Build history of the part. All positions in model axes, mm. A direction names the side the tool comes from. Round coordinates to 2 decimals unless told otherwise and drop trailing zeros. Order: outer loops, then holes, each group sorted by start corner. A loop starts at its lowest first (then second) coordinate and runs counter-clockwise, first axis right, second up. Notation, with made-up numbers: M -25,16.25 L -7,16.25 A22 cw -7,24.25 Z; hole C 7,62 d5. An arc over 180 degrees is marked long. Use CSV: the item, a comma, the result in double quotes.
Autodesk Inventor part; units mm, degrees
ref_plane "YZ Plane" through (0, 0, 0) normal (1, 0, 0) x (0, 1, 0)
ref_plane "XZ Plane" through (0, 0, 0) normal (0, 1, 0) x (-1, 0, 0)
ref_plane "XY Plane" through (0, 0, 0) normal (0, 0, 1) x (1, 0, 0)
sketch "Skizze1" plane through (0, 0, 0) normal (0, 0, 1) x (1, 0, 0)
  line L0 (0, 9.6853) -> (0, -8.6142)
  line L1 (-61.4142, 0) -> (18.4853, 0)
  arc A0 (3.5355, -3.5355) -> (-3.5355, 3.5355) centre (0, 0) ccw
  line L2 (-8.0711, -1) -> (-50, -1)
  line L3 (-50, -1) -> (-50, -6)
  line L4 (-50, -6) -> (1.0711, -6)
  line L5 (3.5355, -3.5355) -> (1.0711, -6)
  line L6 (-8.0711, -1) -> (-3.5355, 3.5355)
  dimension "d1" = 5
  dimension "d2" = 1
  dimension "d3" = 5
  dimension "d21" = 50
  dimension "d22" = 45
extrude "Extrusion1" add sketch "Skizze1" along normal blind 2
sketch "Skizze2" plane through (0, 0, 0) normal (0, 0, 1) x (1, 0, 0)
  point P0 (0, 0)
  point P1 (0, 0)
hole "Bohrung1" at (0, 0, 0) direction (0, 0, 1) diameter 6 end through all
sketch "Skizze5" plane through (-50, -6, 0) normal (-1, 0, 0) x (0, 0, 1)
  line L0 (0, 5) -> (0, 0)
  line L1 (0, 0) -> (2, 0)
  line L2 (2, 5) -> (2, 0)
  line L3 (0, 5) -> (2, 5)
  line L4 (0, 0) -> (2, 0)
  line L5 (0, 0) -> (-2, 2.3835)
  line L6 (-2, 2.3835) -> (-2, 3)
  line L7 (0, 5) -> (0, 0)
  line L8 (0, 0) -> (0, 5)
  line L9 (-2, 3) -> (-4.6, 3)
  line L10 (-4.6, 3) -> (-4.6, 5)
  line L11 (-4.6, 5) -> (0, 5)
  point P0 (0, 6)
  dimension "d23" = 40
  dimension "d28" = 3
  dimension "d29" = 2
  dimension "d30" = 4.6
extrude "Extrusion4" add sketch "Skizze5" against normal blind 5 contours L0 L5 L6 L9 L10 L11
fillet "Rundung1" radius 2 3 edges at (1.0711, -6, 1) (-8.0711, -1, 1) (-50, -6, 1)
sketch "Skizze8" plane through (0, 0, 0) normal (0, 0, -1) x (-1, 0, 0)
  circle A0 centre (0, 0) radius 5
  arc A1 (3.5355, 3.5355) -> (-3.5355, -3.5355) centre (0, 0) ccw
  circle A2 centre (0, 0) radius 3
  circle A3 centre (0, 0) radius 3
  dimension "d41" = 6
extrude "Extrusion7" add sketch "Skizze8" along normal blind 1
sketch "Skizze6" plane through (0, 0, -1) normal (0, 0, -1) x (-1, 0, 0)
  circle A0 centre (0, 0) radius 1.5
  circle A1 centre (0, 0) radius 3
  dimension "d32" = 3
extrude "Extrusion5" [suppressed]
sketch "Skizze7" plane through (0, 0, -12.2) normal (0, 0, -1) x (-1, 0, 0)
  line L0 (0.2, 2) -> (-0.2, 2)
  line L1 (-0.2, 2) -> (-0.2, -2)
  line L2 (-0.2, -2) -> (0.2, -2)
  line L3 (0.2, -2) -> (0.2, 2)
  line L4 (0.2, 2) -> (-0.2, -2) construction
  line L5 (-0.2, 2) -> (0.2, -2) construction
  point P0 (0, 0)
  dimension "d35" = 0.4
  dimension "d36" = 4
extrude "Extrusion6" [suppressed]
sketch "Skizze9" plane through (0, 0, -1) normal (0, 0, -1) x (-1, 0, 0)
  ellipse E0 centre (0, 0) end of major axis (0, -3.3) minor radius 3
  circle A0 centre (0, 0) radius 3 construction
  dimension "d42" = 3.3
  dimension "d43" = 3
extrude "Extrusion8" [suppressed]
chamfer "Fase1" [suppressed]
properties part number "Akkusperre Klein"
(1) Wall check: line 1 (Y direction, x = 0, z = 1.5); line 2 (X direction, y = -4, z = -0.5); line 3 (Z direction, x = -20, y = -1.5). Give the ranges that are in metal, low to high. Write a range as from..to.
Answer block:
line 1,"y = -6..-3, 3..5"
line 2,"x = -50..-45, -3..3"
line 3,"z = 0..2"
(2) Tool access for faces 4 (the face through (-48, -3, -3)), 5 (the face through (-45, -2, -2)), 6 (the face through (-47.54, -4.82, -0.99)): list every direction of +Z, -Z, +X, -X, +Y, -Y with a clear straight run to the whole face (end or side of a thin tool).
Answer block:
face 4,"-Z, +X, -X, -Y"
face 5,"-Z, +Y, -Y"
face 6,"-Z, -X, -Y"
(3) Cut at A-A, the plane z = 1.5. Give the cut face in (x, y).
Answer block:
outline,"M -50,-4 A2 ccw -48,-6 L 0.24,-6 A2 ccw 1.66,-5.41 L 3.54,-3.54 A5 ccw -3.54,3.54 L -7.49,-0.41 A2 cw -8.9,-1 L -50,-1 Z; hole C 0,0 d6"
(4) Cut at D-D, the plane y = 4. Give the cut face in (x, z), and give its area (3 significant figures).
Answer block:
outline,"M -3,-1 L 3,-1 L 3,2 L -3,2 Z"
area,"18.0 mm²"
(5) Cut at C-C, the plane x = -32.5. Give the cut face in (y, z).
Answer block:
outline,"M -6,0 L -1,0 L -1,2 L -6,2 Z"
(6) Cut at B-B, the plane y = 1.25. Give the cut face in (x, z), and give its area (3 significant figures).
Answer block:
outline,"M -5.82,0 L -4.84,0 L -4.84,-1 L -2.73,-1 L -2.73,2 L -5.82,2 Z; M 2.73,-1 L 4.84,-1 L 4.84,2 L 2.73,2 Z"
area,"14.6 mm²"
(7) Two-plate mould, pull along Y, no slides. Class faces 1 (the face through (-49.65, -5.13, 0.6)), 2 (the face through (-21, -3, 0)), 3 (the face through (-1.117, 2.784, 0.521)): released by +Y, released by -Y, zero draft, split by the parting line, or undercut.
Answer block:
face 1,"released by -Y"
face 2,"zero draft"
face 3,"undercut"
(8) Drop flat-ended pins along their axis: pin 1 (5 mm diameter, centred on x = 0, y = -1.5, fed in from -Z); pin 2 (1 mm diameter, centred on x = -17.5, y = -2.5, fed in from -Z); pin 3 (1.4 mm diameter, centred on y = -2.5, z = -1.5, fed in from +X). Give the stop position or say it passes through.
Answer block:
pin 1,"stops at z = -1"
pin 2,"stops at z = 0"
pin 3,"stops at x = 4.58"
